Part model, mm, in its own coordinate system. Face numbers are marked on the shaded views. A direction names the side the tool comes from. Give positions to 0.01 mm unless a question says otherwise; leave off trailing zeros. Order: outer loops, then holes, each group sorted by start corner. A loop starts at its lowest first (then second) coordinate and runs counter-clockwise, first axis right, second up.
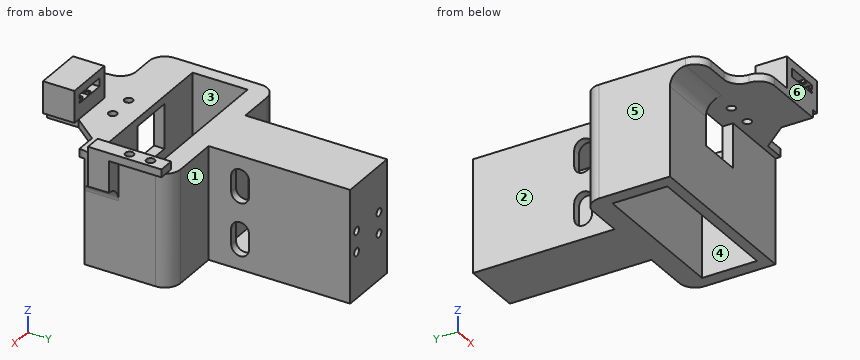
from build123d import *

# Parameters (mm, degrees)
SKETCH_2_W           = 17
SKETCH_2_H           = 17
EXTRUDE_1_DEPTH      = 47
SHELL_2_T            = 3
SKETCH_8_R           = 1.6
SKETCH_8_W           = 56
SKETCH_8_H           = 21
EXTRUDE_2_DEPTH      = 3
SKETCH_9_W           = 66
SKETCH_9_H           = 4
EXTRUDE_3_DEPTH      = 40
SKETCH_11_W          = 13
SKETCH_11_H          = 13
CUT_EXTRUDE_3_DEPTH  = 3
EXTRUDE_START        = -48
SKETCH_13_W          = 17
SKETCH_13_H          = 17
EXTRUDE_4_DEPTH      = 3
SKETCH_17_W          = 17
SKETCH_17_H          = 17
CUT_EXTRUDE_4_DEPTH  = 78.409624725
SKETCH_19_W          = 30
SKETCH_19_H          = 12
EXTRUDE_8_DEPTH      = 3
SKETCH_20_W          = 0.8
SKETCH_20_H          = 1.1
SKETCH_20_W_2        = 2.1
SKETCH_20_H_2        = 0.8
EXTRUDE_9_DEPTH      = 12
FILLET_5_R           = 6
EXTRUDE_11_DEPTH     = 20
EXTRUDE_START_2      = 3
SKETCH_23_W          = 6
SKETCH_23_H          = 28
SKETCH_23_R          = 1.6
EXTRUDE_12_DEPTH     = 3
EXTRUDE_START_3      = -28
SKETCH_24_W          = 6
SKETCH_24_H          = 12
EXTRUDE_13_DEPTH     = 8
FILLET_START         = -40
FILLET_6_DEPTH       = 43
FILLET_START_2       = -6
FILLET_6_2_DEPTH     = 9
FILLET_START_3       = -33
FILLET_6_3_DEPTH     = 13
FILLET_START_4       = -11
FILLET_6_4_DEPTH     = 11
EXTRUDE_START_4      = 12
EXTRUDE_14_DEPTH     = 12
SKETCH_26_W          = 17
SKETCH_26_H          = 29
CUT_EXTRUDE_6_DEPTH  = 50
SKETCH_29_W          = 35
SKETCH_29_H          = 4
EXTRUDE_15_DEPTH     = 23
SKETCH_30_W          = 23
SKETCH_30_H          = 35
EXTRUDE_16_DEPTH     = 10
EXTRUDE_START_5      = 8
EXTRUDE_17_DEPTH     = 8
CUT_EXTRUDE_10_DEPTH = 82.579715616
SKETCH_33_W          = 17
SKETCH_33_H          = 37
CUT_EXTRUDE_11_DEPTH = 44
SKETCH_35_W          = 17
SKETCH_35_H          = 37
EXTRUDE_18_DEPTH     = 3
SKETCH_31_R          = 1.5
CUT_EXTRUDE_13_DEPTH = 5
SKETCH_39_R          = 1.5
CUT_EXTRUDE_14_DEPTH = 1.5


with BuildPart() as part:
    # Sketch 2 → Extrude 1 (new body)
    with BuildSketch(Plane(origin=(0, 0, 0), x_dir=(1, 0, 0), z_dir=(0, 1, 0))):
        with Locations((8.5, 8.5)):
            Rectangle(SKETCH_2_W, SKETCH_2_H)
    extrude(amount=EXTRUDE_1_DEPTH)

    # Shell 2
    shell_2_openings = [part.faces().sort_by_distance(p)[0] for p in [
        (8.5, 0, -8.5),
    ]]
    offset(amount=SHELL_2_T, openings=shell_2_openings, kind=Kind.INTERSECTION)

    # Sketch 8 → Extrude 2 (add)
    with BuildSketch(Plane.XY.offset(3)):
        Polygon((-22.5, 0), (43.5, 0), (43.5, -35), (35.5, -35), (27.5, -45), (-22.5, -45), align=None)
        with Locations((8.5, -37.5)):
            Circle(SKETCH_8_R, mode=Mode.SUBTRACT)
        with Locations((18.5, -37.5)):
            Circle(SKETCH_8_R, mode=Mode.SUBTRACT)
        with Locations((10.5, -18.5)):
            Rectangle(SKETCH_8_W, SKETCH_8_H, mode=Mode.SUBTRACT)
    extrude(amount=-EXTRUDE_2_DEPTH)

    # Sketch 9 → Extrude 3 (add)
    with BuildSketch(Plane(origin=(0, 0, 0), x_dir=(-1, 0, 0), z_dir=(0, 0, -1))):
        with Locations((-10.5, -31)):
            Rectangle(SKETCH_9_W, SKETCH_9_H)
    extrude(amount=EXTRUDE_3_DEPTH)

    # Sketch 11 → Cut-Extrude 3 (cut)
    with BuildSketch(Plane(origin=(0, 50, 0), x_dir=(1, 0, 0), z_dir=(0, 1, 0))):
        with Locations((8.5, 8.5)):
            Rectangle(SKETCH_11_W, SKETCH_11_H)
    extrude(amount=-CUT_EXTRUDE_3_DEPTH, mode=Mode.SUBTRACT)

    # Sketch 13 → Extrude 4 (add)
    with BuildSketch(Plane(origin=(0, 50, 0), x_dir=(1, 0, 0), z_dir=(0, 1, 0)).offset(EXTRUDE_START)):
        with Locations((8.5, 8.5)):
            Rectangle(SKETCH_13_W, SKETCH_13_H)
    extrude(amount=EXTRUDE_4_DEPTH)

    # Sketch 17 → Cut-Extrude 4 (cut, through all)
    with BuildSketch(Plane(origin=(0, 5, 0), x_dir=(1, 0, 0), z_dir=(0, 1, 0))):
        with Locations((8.5, 8.5)):
            Rectangle(SKETCH_17_W, SKETCH_17_H)
    extrude(amount=-CUT_EXTRUDE_4_DEPTH, mode=Mode.SUBTRACT)

    # Sketch 19 → Extrude 8 (add)
    with BuildSketch(Plane.XY.offset(3)):
        with Locations((12.5, -51)):
            Rectangle(SKETCH_19_W, SKETCH_19_H)
    extrude(amount=-EXTRUDE_8_DEPTH)

    # Sketch 20 → Extrude 9 (add)
    # profile 1 of 4: a face of its own
    with BuildSketch(Plane.XZ.offset(57)):
        Polygon((27.5, 3), (30.1, 3), (30.1, 15.1), (11.4, 15.1), (11.4, 3), align=None)
        Polygon((14.4, 8.9), (14.4, 12.1), (22.6, 12.1), (23.4, 12.1), (27.1, 12.1), (27.1, 10.4), (27.1, 9.6), (27.1, 8.9), (20.9, 8.9), (20.1, 8.9), align=None, mode=Mode.SUBTRACT)
    # profile 2 of 4: a face of its own
    with BuildSketch(Plane.XZ.offset(57)):
        with Locations((23, 11.55)):
            Rectangle(SKETCH_20_W, SKETCH_20_H)
    # profile 3 of 4: a face of its own
    with BuildSketch(Plane.XZ.offset(57)):
        with Locations((20.5, 9.45)):
            Rectangle(SKETCH_20_W, SKETCH_20_H)
    # profile 4 of 4: a face of its own
    with BuildSketch(Plane.XZ.offset(57)):
        with Locations((26.05, 10)):
            Rectangle(SKETCH_20_W_2, SKETCH_20_H_2)
    extrude(amount=-EXTRUDE_9_DEPTH)

    # Fillet 5
    fillet_5_edges = [part.edges().sort_by_distance(p)[0] for p in [
        (-11.25, -33, 0),
        (-22.5, -45, 1.5),
        (-2.5, -57, 1.5),
        (-2.5, -45, 1.5),
    ]]
    fillet(fillet_5_edges, radius=FILLET_5_R - 0.0001)  # a hair under: the kernel refuses the full size

    # Sketch 22 → Extrude 11 (add)
    with BuildSketch(Plane(origin=(0, 0, 0), x_dir=(-1, 0, 0), z_dir=(0, 0, -1))):
        Polygon((0, 0), (-17, 0), (-20, 0), (-43.5, 0), (-43.5, -29), (-38.5, -29), (-38.5, -8), (17.5, -8), (17.5, -29), (22.5, -29), (22.5, 0), (3, 0), align=None)
    extrude(amount=EXTRUDE_11_DEPTH)



with BuildPart() as body_2:
    # Sketch 23 → Extrude 12 (new body)
    with BuildSketch(Plane.XY.offset(3).offset(EXTRUDE_START_2)):
        with Locations((46.5, -14)):
            Rectangle(SKETCH_23_W, SKETCH_23_H)
        with Locations((46.5, -6)):
            Circle(SKETCH_23_R, mode=Mode.SUBTRACT)
        with Locations((46.5, -14)):
            Circle(SKETCH_23_R, mode=Mode.SUBTRACT)
    extrude(amount=EXTRUDE_12_DEPTH)


with BuildPart() as part_1:
    add(part.part)

    add(body_2.part)  # Extrude 13 merges body 2
    # Sketch 24 → Extrude 13 (add)
    with BuildSketch(Plane(origin=(0, 0, 0), x_dir=(1, 0, 0), z_dir=(0, 1, 0)).offset(EXTRUDE_START_3)):
        with Locations((46.5, 0)):
            Rectangle(SKETCH_24_W, SKETCH_24_H)
    extrude(amount=EXTRUDE_13_DEPTH)

    # Fillet 6: read off the stored shape, not the designer's step
    # Fillet 6 outline → Fillet 6 (cut)
    with BuildSketch(Plane.XY.offset(FILLET_START)):
        with BuildLine():
            ThreePointArc((37.5, 0), (41.742640687, -1.757359313), (43.5, -6))
            Line((43.5, -6), (43.5, 0))
            Line((43.5, 0), (37.5, 0))
        make_face()
        with BuildLine():
            Line((-22.5, 0), (-22.5, -6))
            ThreePointArc((-22.5, -6), (-20.742640687, -1.757359313), (-16.5, 0))
            Line((-16.5, 0), (-22.5, 0))
        make_face()
    extrude(amount=FILLET_6_DEPTH, mode=Mode.SUBTRACT)

    # Fillet 6 2 outline → Fillet 6 2 (add)
    with BuildSketch(Plane.XY.offset(FILLET_START_2)):
        with BuildLine():
            Line((43.5, -28), (43.5, -34))
            ThreePointArc((43.5, -34), (45.257359313, -29.757359313), (49.5, -28))
            Line((49.5, -28), (43.5, -28))
        make_face()
    extrude(amount=FILLET_6_2_DEPTH)

    # Fillet 6 3 outline → Fillet 6 3 (add)
    with BuildSketch(Plane(origin=(0, 0, 0), x_dir=(1, 0, 0), z_dir=(0, 1, 0)).offset(FILLET_START_3)):
        with BuildLine():
            ThreePointArc((49.5, 6), (45.257359313, 7.757359313), (43.5, 12))
            Line((43.5, 12), (43.5, 6))
            Line((43.5, 6), (49.5, 6))
        make_face()
    extrude(amount=FILLET_6_3_DEPTH)

    # Fillet 6 4 outline → Fillet 6 4 (cut)
    with BuildSketch(Plane.XY.offset(FILLET_START_4)):
        with BuildLine():
            ThreePointArc((49.5, -28), (45.627016654, -29.417424305), (43.583920217, -33))
            Line((43.583920217, -33), (49.5, -33))
            Line((49.5, -33), (49.5, -28))
        make_face()
        with BuildLine():
            ThreePointArc((43.5, -34), (43.521016863, -33.498242438), (43.583920217, -33))
            Line((43.583920217, -33), (43.5, -33))
            Line((43.5, -33), (43.5, -34))
        make_face()
    extrude(amount=FILLET_6_4_DEPTH, mode=Mode.SUBTRACT)

    # Sketch 25 → Extrude 14 (add)
    with BuildSketch(Plane(origin=(0, 0, -20), x_dir=(-1, 0, 0), z_dir=(0, 0, -1)).offset(EXTRUDE_START_4)):
        with BuildLine():
            Line((22.5, -29), (22.5, -6))
            ThreePointArc((22.5, -6), (20.742640687, -1.757359313), (16.5, 0))
            Line((16.5, 0), (3, 0))
            Line((3, 0), (3, 50))
            Line((3, 50), (-20, 50))
            Line((-20, 50), (-20, 0))
            Line((-20, 0), (-37.5, 0))
            ThreePointArc((-37.5, 0), (-41.742640687, -1.757359313), (-43.5, -6))
            Line((-43.5, -6), (-43.5, -29))
            Line((-43.5, -29), (-38.5, -29))
            Line((-38.5, -29), (-38.5, -8))
            Line((-38.5, -8), (17.5, -8))
            Line((17.5, -8), (17.5, -29))
            Line((17.5, -29), (22.5, -29))
        make_face()
    extrude(amount=-EXTRUDE_14_DEPTH)

    # Sketch 26 → Cut-Extrude 6 (cut)
    with BuildSketch(Plane(origin=(0, 50, 0), x_dir=(1, 0, 0), z_dir=(0, 1, 0))):
        with Locations((8.5, 14.5)):
            Rectangle(SKETCH_26_W, SKETCH_26_H)
    extrude(amount=-CUT_EXTRUDE_6_DEPTH, mode=Mode.SUBTRACT)

    # Sketch 29 → Extrude 15 (add)
    with BuildSketch(Plane(origin=(20, 0, 0), x_dir=(0, 0, -1), z_dir=(1, 0, 0))):
        with Locations((14.5, 52)):
            Rectangle(SKETCH_29_W, SKETCH_29_H)
    extrude(amount=-EXTRUDE_15_DEPTH)

    # Sketch 30 → Extrude 16 (add)
    with BuildSketch(Plane(origin=(0, 54, 0), x_dir=(1, 0, 0), z_dir=(0, 1, 0))):
        with Locations((8.5, 14.5)):
            Rectangle(SKETCH_30_W, SKETCH_30_H)
    extrude(amount=-EXTRUDE_16_DEPTH)

    # Sketch 32 → Extrude 17 (add)
    with BuildSketch(Plane(origin=(0, 0, -32), x_dir=(-1, 0, 0), z_dir=(0, 0, -1)).offset(EXTRUDE_START_5)):
        with BuildLine():
            Line((-20, 0), (-37.5, 0))
            ThreePointArc((-37.5, 0), (-41.742640687, -1.757359313), (-43.5, -6))
            Line((-43.5, -6), (-43.5, -29))
            Line((-43.5, -29), (-38.5, -29))
            Line((-38.5, -29), (-38.5, -8))
            Line((-38.5, -8), (17.5, -8))
            Line((17.5, -8), (17.5, -29))
            Line((17.5, -29), (22.5, -29))
            Line((22.5, -29), (22.5, -6))
            ThreePointArc((22.5, -6), (20.742640687, -1.757359313), (16.5, 0))
            Line((16.5, 0), (3, 0))
            Line((3, 0), (3, 54))
            Line((3, 54), (-20, 54))
            Line((-20, 54), (-20, 0))
        make_face()
    extrude(amount=-EXTRUDE_17_DEPTH)

    # Sketch 34 → Cut-Extrude 10 (cut, through all)
    with BuildSketch(Plane(origin=(20, 0, 0), x_dir=(0, 0, -1), z_dir=(1, 0, 0))):
        with BuildLine():
            Line((5.5, 15.4), (11.5, 15.4))
            ThreePointArc((11.5, 15.4), (14.9, 12), (11.5, 8.6))
            Line((11.5, 8.6), (5.5, 8.6))
            ThreePointArc((5.5, 8.6), (2.1, 12), (5.5, 15.4))
        make_face()
        with BuildLine():
            Line((25.5, 15.4), (31.5, 15.4))
            ThreePointArc((31.5, 15.4), (34.9, 12), (31.5, 8.6))
            Line((31.5, 8.6), (25.5, 8.6))
            ThreePointArc((25.5, 8.6), (22.1, 12), (25.5, 15.4))
        make_face()
    extrude(amount=-CUT_EXTRUDE_10_DEPTH, mode=Mode.SUBTRACT)

    # Sketch 33 → Cut-Extrude 11 (cut)
    with BuildSketch(Plane(origin=(0, 0, 0), x_dir=(1, 0, 0), z_dir=(0, 1, 0))):
        with Locations((8.5, 18.5)):
            Rectangle(SKETCH_33_W, SKETCH_33_H)
    extrude(amount=CUT_EXTRUDE_11_DEPTH, mode=Mode.SUBTRACT)

    # Sketch 35 → Extrude 18 (add)
    with BuildSketch(Plane(origin=(0, 0, 0), x_dir=(1, 0, 0), z_dir=(0, 1, 0))):
        with Locations((8.5, 18.5)):
            Rectangle(SKETCH_35_W, SKETCH_35_H)
    extrude(amount=EXTRUDE_18_DEPTH)

    # Sketch 31 → Cut-Extrude 13 (cut)
    with BuildSketch(Plane(origin=(0, 54, 0), x_dir=(1, 0, 0), z_dir=(0, 1, 0))):
        with Locations(Location((2, 22.5, 0), (0, 0, 270))):
            Circle(SKETCH_31_R)
        with Locations(Location((2, 14.5, 0), (0, 0, 270))):
            Circle(SKETCH_31_R)
        with Locations(Location((16, 22.5, 0), (0, 0, 270))):
            Circle(SKETCH_31_R)
        with Locations(Location((16, 14.5, 0), (0, 0, 270))):
            Circle(SKETCH_31_R)
    extrude(amount=-CUT_EXTRUDE_13_DEPTH, mode=Mode.SUBTRACT)

    # Sketch 39 → Cut-Extrude 14 (cut)
    with BuildSketch(Plane(origin=(0, 49, 0), x_dir=(1, 0, 0), z_dir=(0, 1, 0))):
        with Locations(Location((2, 14.5, 0), (0, 0, 270))):
            Circle(SKETCH_39_R)
        with Locations(Location((16, 22.5, 0), (0, 0, 270))):
            Circle(SKETCH_39_R)
    extrude(amount=-CUT_EXTRUDE_14_DEPTH, mode=Mode.SUBTRACT)


solid = part_1.part
Item 1: Band-saw the part on A-A on y = 12. List the corners of the cut face in (x, z), plus the area to 3 significant figures.
Item 2: Which spindle directions (+Z, -Z, +X, -X, +Y, -Y) get a long thin tool onto all of the face, cutting with end or side? Do the marked faces 1, 2 and 3. Say none if no direction does.
Item 3: Band-saw the part on D-D on y = 32.5. List the corners of the cut face in (x, z).
Item 4: Pull direction X, two halves, no side cores. Call the marked faces 4, 5 and 6: released by +X, released by -X, zero draft, split by the parting line, or undercut.
Item 5: Drop flat-ended pins along their axis: P1, Ø8.5, axis at x = -1, y = -36.5, coming from the -Z side; P2, Ø3.5, axis at x = 18.5, y = -37.5, coming from the +Z side; P3, Ø2.5, axis at x = -1, z = -29.5, coming from the -Y side; P4, Ø3.5, axis at x = 39, z = 1, coming from the -Y side. Give the stop position or say it passes through.
Item 6: Band-saw the part on B-B on x = 5.5. List the corners of the cut face in (y, z).
Item 7: Band-saw the part on C-C on x = -14.5. List the corners of the cut face in (y, z).
Item 8: Drill centre lines: probe 1 along Y at (x, z) = (18.5, 2.1); probe 2 along Y at (x, z) = (19.5, -9); probe 3 along X at (y, z) = (52.25, -14.5). Where is each one in solid material? Low to high.
Working result:
1. outline: (-3, -40) - (20, -40) - (20, -34.9) - (17, -34.9) - (17, -37) - (0, -37) - (0, -34.9) - (-3, -34.9) - close; (-3, -22.1) - (0, -22.1) - (0, -14.9) - (-3, -14.9) - close; (-3, -2.1) - (0, -2.1) - (0, 0) - (17, 0) - (17, -2.1) - (20, -2.1) - (20, 3) - (-3, 3) - close; (17, -22.1) - (20, -22.1) - (20, -14.9) - (17, -14.9) - close
1. area: 206 mm2
2. face 1: +Z, -Z, +X, +Y
2. face 2: +Z, -Z, -X, +Y
2. face 3: +Z, -Z
3. outline: (-3, -40) - (20, -40) - (20, 3) - (-3, 3) - close; hole (0, -37) - (17, -37) - (17, 0) - (0, 0) - close
4. face 4: undercut
4. face 5: released by -X
4. face 6: zero draft
5. P1: stops at z = -40
5. P2: stops at z = 3
5. P3: stops at y = -33
5. P4: stops at y = -35
6. outline: (-57, 0) - (-29, 0) - (-29, 3) - (-57, 3) - close; (-33, -40) - (-29, -40) - (-29, -17) - (-33, -17) - close; (-8, -40) - (54, -40) - (54, 3) - (-8, 3) - close; hole (3, -37) - (44, -37) - (44, 0) - (3, 0) - close
7. outline: (-45, 0) - (-39, 0) arc R6 cw to (-33, -6) - (-33, -40) - (-29, -40) - (-29, 3) - (-45, 3) - close; (-8, -40) - (0, -40) - (0, 3) - (-8, 3) - close
8. probe 1: y = -57 to -39.1, -35.9 to -29, -8 to 54
8. probe 2: y = -33 to -29, -8 to 8.6, 15.4 to 54
8. probe 3: x = -3 to 0.5, 3.5 to 14.5, 17.5 to 20
